```python
from build123d import *

# Parameters (mm, degrees)
BASPROSKE_W     = 12
BASPROSKE_H     = 6.3
TOOTHCUT_DEPTH  = 15.945902448
TEETHCUTS_COUNT = 12
TEETHCUTS_ANGLE = 330
BORE_DEPTH      = 50.0000508


with BuildPart() as part:
    # BasProSke → Base-Revolve (revolve)
    with BuildSketch(Plane(origin=(0, 0, 0), x_dir=(1, 0, 0), z_dir=(0, 1, 0)), mode=Mode.PRIVATE) as base_revolve_sk:
        with Locations((6, 3.15)):
            Rectangle(BASPROSKE_W, BASPROSKE_H)
    revolve(base_revolve_sk.sketch.rotate(Axis((-10, 0, 0), (1, 0, 0)), 180), axis=Axis((-10, 0, 0), (1, 0, 0)))

    # TooCutSke → ToothCut (cut, through all)
    with BuildSketch(Plane(origin=(0, 0, 0), x_dir=(0, 0, -1), z_dir=(1, 0, 0))):
        with BuildLine():
            ThreePointArc((0.505712998, 4.243975773), (0, 4.274), (-0.505712998, 4.243975773))
            ThreePointArc((-0.505712998, 4.243975773), (-0.754225381, 5.326869831), (-1.508135905, 6.142980649))
            ThreePointArc((-1.508135905, 6.142980649), (0, 6.3254), (1.508135905, 6.142980649))
            ThreePointArc((1.508135905, 6.142980649), (0.754225381, 5.326869831), (0.505712998, 4.243975773))
        make_face()
    toothcut = extrude(amount=TOOTHCUT_DEPTH, mode=Mode.SUBTRACT)

    # TeethCuts: ToothCut ×12 about axis
    teethcuts_axis = Axis((-10, 0, 0), (1, 0, 0))
    for i in range(1, TEETHCUTS_COUNT):
        add(toothcut.rotate(teethcuts_axis, i * TEETHCUTS_ANGLE / (TEETHCUTS_COUNT - 1)), mode=Mode.SUBTRACT)

    # BorSke → Bore (cut, symmetric)
    with BuildSketch(Plane(origin=(0, 0, 0), x_dir=(0, 0, -1), z_dir=(1, 0, 0))):
        with BuildLine():
            Line((-1.483239697, 1.95), (1.483239697, 1.95))
            ThreePointArc((1.483239697, 1.95), (0, -2.45), (-1.483239697, 1.95))
        make_face()
    extrude(amount=BORE_DEPTH, both=True, mode=Mode.SUBTRACT)


solid = part.part
```
Here's how the part is built. I have some questions about the finished solid (model axes, mm). A direction names the side the tool comes from. Give positions to 0.01 mm unless a question says otherwise; leave off trailing zeros. Loops run counter-clockwise (first coordinate to the right, second up) from the corner with the lowest first, then second, coordinate; pieces in that order, holes last. Notation, with made-up numbers: M -28,74.25 L 9,74.25 A24 ccw 9,101.25 Z; hole C -23,79 d7. An arc over 180 degrees is marked long. Put each result on its own line as item: value. Start each with the question number.
(1) I need wall thicknesses on line 1 along Z through (x, y) = (5.5, 1); line 2 along Z through (x, y) = (4, 3.75); line 3 along Y through (x, z) = (11.25, 5). Which ranges of each line are inside material? Lowest first, please. Write a range as [from, to].
(2) I want a section at C-C on z = -3.75. Please give me the cut outline in (x, y), then the cut area to 3 significant figures.
(3) For faces 1 (the flat face through (0, 0, -3)), 2 (the cylindrical face through (5.916, 3.315, 4.235)), which set-ups out of +Z, -Z, +X, -X, +Y, -Y let a thin tool reach every point of the face, with its end or its side?
(4) If we mould it in two halves opening along Z, with no side actions, what happens to faces 3 (the cylindrical face through (5.92, -4.99, -2.01)), 4 (the flat face through (12, 0, 3))? For each: +Z half, -Z half, draft (parallel to the pull), parting line (faces both ways), or undercut.
(5) I want a section at B-B on y = 0. Please give me the cut outline in (x, z).
(6) Will these pins go through, and if not, where does the flat tip stop? pin 1 Ø1 at (x, y) = (5.5, 3.5) entering from -Z; pin 2 Ø1.5 at (x, y) = (8.5, -4.5) entering from +Z; pin 3 Ø0.9 at (x, z) = (5.5, -0.5) entering from -Y.
(7) I want a section at A-A on z = 0. Please give me the cut outline in (x, y), then the cut area to 3 significant figures.
Answer block:
1. line 1: [-5.7, -2.24], [2.24, 5.7]
1. line 2: [-4.45, -2.77], [-2.05, 2.05], [2.77, 4.45]
1. line 3: [-2.01, -0.61], [0.61, 2.01]
2. outline: M 0,-4.45 L 12,-4.45 L 12,-2.77 L 0,-2.77 Z; M 0,-2.05 L 12,-2.05 L 12,2.05 L 0,2.05 Z; M 0,2.77 L 12,2.77 L 12,4.45 L 0,4.45 Z
2. area: 89.3 mm^2
3. face 1: +Z, -Z, -X, +Y, -Y
3. face 2: +Z, +X, -X
4. face 3: undercut
4. face 4: draft
5. outline: M 0,-4.27 L 12,-4.27 L 12,-2.45 L 0,-2.45 Z; M 0,2.45 L 12,2.45 L 12,4.27 L 0,4.27 Z
6. pin 1: z = -4.52
6. pin 2: z = 4.56
6. pin 3: y = -5.63
7. outline: M 0,-4.27 L 12,-4.27 L 12,-2.45 L 0,-2.45 Z; M 0,1.95 L 12,1.95 L 12,4.27 L 0,4.27 Z
7. area: 49.8 mm^2
